Source: three-view drawing plus pictorial views. Frame: mm from the lowest corner of the part. Give positions to 0.01 mm unless a question says otherwise; leave off trailing zeros. Order: outer loops, then holes, each group sorted by start corner. A loop starts at its lowest first (then second) coordinate and runs counter-clockwise, first axis right, second up. Notation, with made-up numbers: M 52.25,63.5 L 72.25,63.5 A34 ccw 72.25,96.5 Z; hole C 85.25,6.25 d3. An arc over 180 degrees is marked long. One line per question, with ' | ' between items. Start each with the question number.
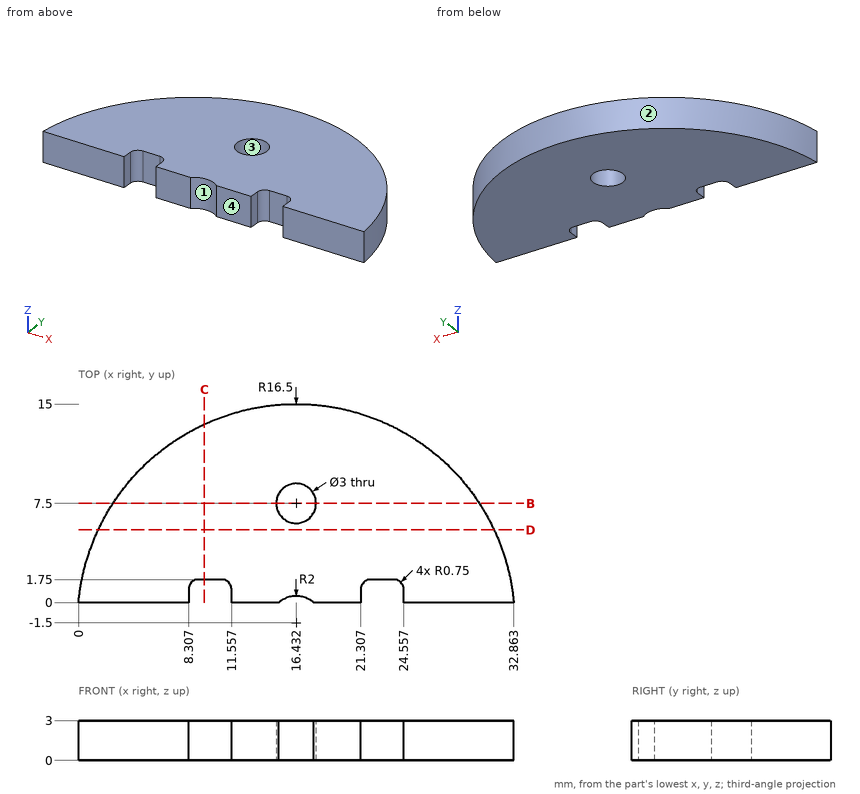
Item 1: Cut plane B-B on y = 7.5. Return the cut outline in (x, z).
Item 2: Cut plane C-C on x = 9.5. Return the cut outline in (y, z).
Item 3: Mould query, pull axis X, two halves, no side actions, for the marked faces 1, 2, 3 and 4. Classes: pulls with the +X half, pulls with the -X half, needs draft (parallel to the pull), parting line crosses it, or undercut.
Item 4: Pin query (flat end, axial travel): pin 1 Ø1 at (x, z) = (5.5, 1.5) entering from +Y (1 decimal); pin 2 Ø2 at (x, y) = (29.5, 11) entering from -Z; pin 3 Ø1.4 at (x, z) = (10, 1.5) entering from -Y; pin 4 Ø0.5 at (y, z) = (0.5, 2) entering from -X (1 decimal). Return the tip coordinate at first contact, or that it passes through.
Item 5: Cut plane D-D on y = 5.5. Return the cut outline in (x, z).
Item 6: Line query: line 1 (X direction, y = 1.5, z = 1.65) (1 decimal); line 2 (X direction, y = 7.5, z = 2.2); line 3 (X direction, y = 6.75, z = 2.85). Output: solid intervals per line, ascending.
Results are:
1) outline: M 2.6,0 L 14.93,0 L 14.93,3 L 2.6,3 Z; M 17.93,0 L 30.26,0 L 30.26,3 L 17.93,3 Z
2) outline: M 1.75,0 L 13.47,0 L 13.47,3 L 1.75,3 Z
3) face 1: undercut | face 2: parting line crosses it | face 3: undercut | face 4: needs draft
4) pin 1: stops at y = 11.3 | pin 2: passes through | pin 3: stops at y = 1.75 | pin 4: stops at x = 0
5) outline: M 1.49,0 L 31.37,0 L 31.37,3 L 1.49,3 Z
6) line 1: x = 0.2 to 8.5, 11.4 to 21.5, 24.4 to 32.7 | line 2: x = 2.6 to 14.93, 17.93 to 30.26 | line 3: x = 2.14 to 15.13, 17.73 to 30.72
